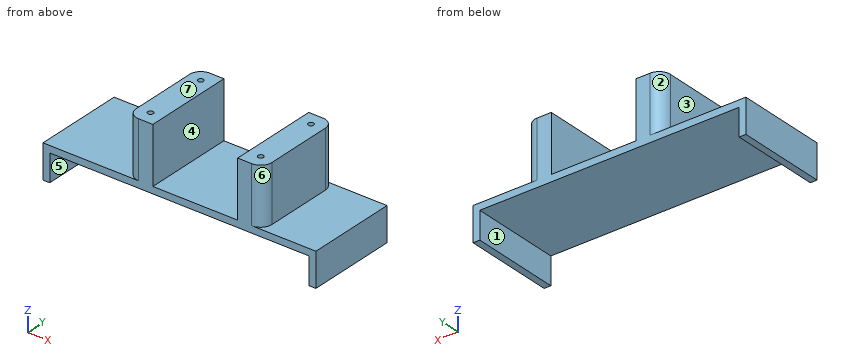
from build123d import *

# Parameters (mm, degrees)
F1_DEPTH = 40
F2_W     = 11.2577080727
F2_H     = 40
F2_W_2   = 11.2422919273
F3_DEPTH = 25
F5_D     = 2.4
F5_DEPTH = 10
F5_TIP   = 0.7210327428
F6_R     = 5


with BuildPart() as f1:
    # F0 (on Front) → F1 (new body)
    with BuildSketch(Plane.XZ):
        Polygon((60.35, 15), (-60.35, 15), (-60.35, 0), (-57.35, 0), (-57.35, 12), (57.35, 12), (57.35, 0), (60.35, 0), align=None)
    extrude(amount=F1_DEPTH)

    # F2 (on face) → F3 (join)
    with BuildSketch(Plane.XY.offset(15)):
        with Locations((-17.4, -20)):
            Rectangle(F2_W, F2_H)
        with Locations((31.35, -20)):
            Rectangle(F2_W_2, F2_H)
    extrude(amount=F3_DEPTH)

    # F5
    with Locations(Plane.XY.offset(40)):
        with Locations((-17.4, -5.875), (31.35, -5.875), (31.35, -34.125), (-17.4, -34.125)):
            Hole(F5_D / 2, depth=F5_DEPTH)
            with Locations((0, 0, -(F5_DEPTH + F5_TIP / 2))):  # 118° drill point
                Cone(0, F5_D / 2, F5_TIP, mode=Mode.SUBTRACT)

    # F6
    f6_edges = [f1.edges().sort_by_distance(p)[0] for p in [
        (-23.028854, 0, 27.5),
        (36.971146, 0, 27.5),
        (36.971146, -40, 27.5),
        (-23.028854, -40, 27.5),
    ]]
    fillet(f6_edges, radius=F6_R)


solid = f1.part
Design review of the part built by this model. Coordinates are the model's own, in mm. Face numbers are marked on the shaded views. A direction names the side the tool comes from. Coordinates: 2 decimals unless noted, no trailing zeros. Loops run counter-clockwise (first coordinate to the right, second up) from the corner with the lowest first, then second, coordinate; pieces in that order, holes last. Notation, with made-up numbers: (25, -39) -> (84, -39) arc R17 cw to (84, -9) -> close; hole circle Ø4 at (89.25, -15.5). An arc over 180 degrees is marked (long way). Use a Markdown table: item, result. Add a question column.
Item 1: Machinability: for the marked faces 1, 2, 3 and 4, which of the approach directions +Z, -Z, +X, -X, +Y, -Y give a long, thin tool a straight path to every point of the face, cutting with its end or side? Answer none if there is none.
Item 2: We need section B-B, the plane y = -8.5. Write out the cut boundary in (x, z), and give its area (3 significant figures).
Item 3: We need section C-C, the plane z = 35.5. Write out the cut boundary in (x, y) (3 decimals).
Item 4: We need section D-D, the plane x = -5.5. Write out the cut boundary in (y, z), and give its area (3 significant figures).
Item 5: The part is to be moulded in two halves that separate along X. For the marked faces 5, 6 and 7, say which applies: +X half, -X half, draft (parallel to the pull), parting line (faces both ways), or undercut.
Item 6: We need section A-A, the plane z = 6. Write out the cut boundary in (x, y).
Item 7: Wall thickness on L1, parallel to Y at x = -17.4, z = 36.5 (3 decimals); L2, parallel to X at y = -17, z = 21; L3, parallel to X at y = -11.5, z = 3: over which ranges is each line inside the solid? List them lowest first. Write a range as from..to.
Item 8: Clearance check with flat-ended pins moving along their axes: P1, Ø12.5, axis at y = -17, z = 23.5, coming from the +X side; P2, Ø12.5, axis at y = -20, z = 23, coming from the -X side; P3, Ø12, axis at x = -4, y = -20, coming from the -Z side; P4, Ø10, axis at x = -42, z = 5.5, coming from the +Y side (3 decimals). State where each tip first meets the part, or that it passes through.
Numbers:
| question | item | result |
|---|---|---|
| 1 | face 1 | -Z, +Y, -Y |
| 1 | face 2 | +Z, -X, +Y |
| 1 | face 3 | +Z, -X, +Y, -Y |
| 1 | face 4 | +Z, +Y, -Y |
| 2 | outline | (-60.35, 0) -> (-57.35, 0) -> (-57.35, 12) -> (57.35, 12) -> (57.35, 0) -> (60.35, 0) -> (60.35, 15) -> (36.97, 15) -> (36.97, 40) -> (25.73, 40) -> (25.73, 15) -> (-11.77, 15) -> (-11.77, 40) -> (-23.03, 40) -> (-23.03, 15) -> (-60.35, 15) -> close |
| 2 | area | 997 mm^2 |
| 3 | outline | (-23.029, -35) arc R5 ccw to (-18.029, -40) -> (-11.771, -40) -> (-11.771, 0) -> (-18.029, 0) arc R5 ccw to (-23.029, -5) -> close; (25.729, -40) -> (31.971, -40) arc R5 ccw to (36.971, -35) -> (36.971, -5) arc R5 ccw to (31.971, 0) -> (25.729, 0) -> close; hole circle Ø2.4 at (-17.4, -34.125); hole circle Ø2.4 at (-17.4, -5.875); hole circle Ø2.4 at (31.35, -34.125); hole circle Ø2.4 at (31.35, -5.875) |
| 4 | outline | (-40, 12) -> (0, 12) -> (0, 15) -> (-40, 15) -> close |
| 4 | area | 120 mm^2 |
| 5 | face 5 | undercut |
| 5 | face 6 | +X half |
| 5 | face 7 | draft |
| 6 | outline | (-60.35, -40) -> (-57.35, -40) -> (-57.35, 0) -> (-60.35, 0) -> close; (57.35, -40) -> (60.35, -40) -> (60.35, 0) -> (57.35, 0) -> close |
| 7 | L1 | y = -40..-35.325, -32.925..-7.075, -4.675..0 |
| 7 | L2 | x = -23.03..-11.77, 25.73..36.97 |
| 7 | L3 | x = -60.35..-57.35, 57.35..60.35 |
| 8 | P1 | stops at x = 36.97 |
| 8 | P2 | stops at x = -23.03 |
| 8 | P3 | stops at z = 12 |
| 8 | P4 | passes through |
